Autodesk Inventor part; units mm, degrees
ref_plane "YZ Plane" through (0, 0, 0) normal (1, 0, 0) x (0, 1, 0)
ref_plane "XZ Plane" through (0, 0, 0) normal (0, 1, 0) x (-1, 0, 0)
ref_plane "XY Plane" through (0, 0, 0) normal (0, 0, 1) x (1, 0, 0)
sketch "Sketch1" plane through (0, 0, 0) normal (0, 0, 1) x (1, 0, 0)
  circle A0 centre (0, 0) radius 200
  line L0 (0, 187.7709) -> (15, 187.7709)
  line L1 (15, 187.7709) -> (15, 182.7709)
  line L2 (15, 182.7709) -> (50, 182.7709)
  line L3 (50, 182.7709) -> (50, 147.7709)
  line L4 (50, 147.7709) -> (-50, 147.7709)
  line L5 (-50, 147.7709) -> (-50, 182.7709)
  line L6 (-50, 182.7709) -> (-15, 182.7709)
  line L7 (-15, 182.7709) -> (-15, 187.7709)
  line L8 (-15, 187.7709) -> (0, 187.7709)
  line L9 (-162.6144, -93.8855) -> (-170.1144, -80.8951)
  line L10 (-170.1144, -80.8951) -> (-165.7843, -78.3951)
  line L11 (-165.7843, -78.3951) -> (-183.2843, -48.0842)
  line L12 (-183.2843, -48.0842) -> (-152.9734, -30.5842)
  line L13 (-152.9734, -30.5842) -> (-102.9734, -117.1867)
  line L14 (-102.9734, -117.1867) -> (-133.2843, -134.6867)
  line L15 (-133.2843, -134.6867) -> (-150.7843, -104.3758)
  line L16 (-150.7843, -104.3758) -> (-155.1144, -106.8758)
  line L17 (-155.1144, -106.8758) -> (-162.6144, -93.8855)
  line L18 (162.6144, -93.8855) -> (155.1144, -106.8758)
  line L19 (155.1144, -106.8758) -> (150.7843, -104.3758)
  line L20 (150.7843, -104.3758) -> (133.2843, -134.6867)
  line L21 (133.2843, -134.6867) -> (102.9734, -117.1867)
  line L22 (102.9734, -117.1867) -> (152.9734, -30.5842)
  line L23 (152.9734, -30.5842) -> (183.2843, -48.0842)
  line L24 (183.2843, -48.0842) -> (165.7843, -78.3951)
  line L25 (165.7843, -78.3951) -> (170.1144, -80.8951)
  line L26 (170.1144, -80.8951) -> (162.6144, -93.8855)
  line L27 (12.5, 183.7364) -> (12.5, 193.7364)
  line L28 (-173.6251, 83.379) -> (-162.3777, 105.706)
  line L29 (-162.3777, 105.706) -> (-153.4469, 101.2071)
  line L30 (-153.4469, 101.2071) -> (-164.6943, 78.88)
  line L31 (-164.6943, 78.88) -> (-173.6251, 83.379)
  line L32 (-181.8421, 26.8753) -> (-182.5998, 1.8868)
  line L33 (-192.5952, 2.1899) -> (-191.8375, 27.1784)
  line L34 (-182.5998, 1.8868) -> (-192.5952, 2.1899)
  line L35 (-191.8375, 27.1784) -> (-181.8421, 26.8753)
  line L36 (-115.9276, 141.0924) -> (-122.1203, 148.9442)
  line L37 (-96.2982, 156.5742) -> (-115.9276, 141.0924)
  line L38 (-102.4909, 164.426) -> (-96.2982, 156.5742)
  line L39 (-122.1203, 148.9442) -> (-102.4909, 164.426)
  line L40 (72.3815, -179.7253) -> (67.6463, -170.9175)
  line L41 (67.6463, -170.9175) -> (89.6659, -159.0795)
  line L42 (94.4011, -167.8873) -> (72.3815, -179.7253)
  line L43 (89.6659, -159.0795) -> (94.4011, -167.8873)
  line L44 (14.035, -182.0694) -> (14.6042, -192.0532)
  line L45 (-10.9244, -183.4924) -> (14.035, -182.0694)
  line L46 (-10.3552, -193.4762) -> (-10.9244, -183.4924)
  line L47 (14.6042, -192.0532) -> (-10.3552, -193.4762)
  line L48 (-64.2258, -170.9424) -> (-67.9293, -180.2313)
  line L49 (-87.4482, -161.6838) -> (-64.2258, -170.9424)
  line L50 (-67.9293, -180.2313) -> (-91.1516, -170.9727)
  line L51 (-91.1516, -170.9727) -> (-87.4482, -161.6838)
  line L52 (119.4559, 152.5469) -> (114.1957, 144.0422)
  line L53 (114.1957, 144.0422) -> (92.9339, 157.1927)
  line L54 (98.1941, 165.6974) -> (119.4559, 152.5469)
  line L55 (92.9339, 157.1927) -> (98.1941, 165.6974)
  line L56 (150.6592, 103.1894) -> (159.0209, 108.6742)
  line L57 (164.3713, 82.2854) -> (150.6592, 103.1894)
  line L58 (172.7329, 87.7702) -> (164.3713, 82.2854)
  line L59 (159.0209, 108.6742) -> (172.7329, 87.7702)
  line L60 (180.1534, 29.85) -> (190.0496, 31.2872)
  line L61 (183.7463, 5.1095) -> (180.1534, 29.85)
  line L62 (190.0496, 31.2872) -> (193.6425, 6.5467)
  line L63 (193.6425, 6.5467) -> (183.7463, 5.1095)
  point P0 (-163.536, 92.293)
  point P1 (-187.2187, 14.5326)
  point P2 (-109.2092, 152.7592)
  point P3 (81.0237, -169.4024)
  point P4 (1.8399, -187.7728)
  point P5 (-77.6887, -170.9575)
  point P6 (106.1949, 154.8698)
  point P7 (161.6961, 95.4798)
  point P8 (186.8979, 18.1984)
  dimension "d12" = 360
  dimension "d28" = 25
  dimension "d32" = 25
  dimension "d36" = 360
extrude "Extrusion1" add sketch "Sketch1" along normal blind 1.5
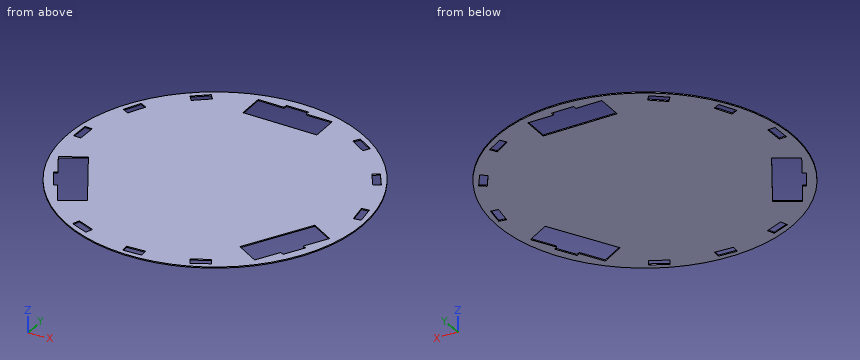
Could you check a few things on this model? Use its own coordinates, in mm. Coordinates: 2 decimals unless noted, no trailing zeros. Order: outer loops, then holes, each group sorted by start corner. A loop starts at its lowest first (then second) coordinate and runs counter-clockwise, first axis right, second up.
Q1. Please list where these lines run through material, in increasing order: L1, parallel to X at y = 84.5, z = 0.1; L2, parallel to X at y = -44, z = 0.9; L3, parallel to Y at x = 108.5, z = 0.95.
Q2. Suppose I cut it at B-B on y = -43. Please give me the cut outline in (x, z).
Q3. Suppose I cut it at C-C on x = 40. Please give me the cut outline in (y, z).
Q4. Will this pin go through, and if not, where does the flat tip stop? pin 1 (0.8 mm diameter, centred on y = 169.5, z = 0.5, fed in from +X).
Q5. Suppose I cut it at D-D on z = 0.5. Give the number of separate pieces and of enclosed holes in the cut face, and give its area (3 significant figures).
Q6. Suppose I cut it at A-A on x = -33.5. Please give me the cut outline in (y, z), and give its area (3 significant figures).
Answer:
1. L1: x = -181.27 to -173.06, -161.86 to 162.92, 167.75 to 181.27
1. L2: x = -195.1 to -176.21, -145.23 to 145.23, 176.21 to 195.1
1. L3: y = -168.01 to -120.38, -107.61 to 147.57, 159.32 to 168.01
2. outline: (-195.32, 0) - (-174.48, 0) - (-174.48, 1.5) - (-195.32, 1.5) - close; (-145.81, 0) - (145.81, 0) - (145.81, 1.5) - (-145.81, 1.5) - close; (174.48, 0) - (195.32, 0) - (195.32, 1.5) - (174.48, 1.5) - close
3. outline: (-195.96, 0) - (147.77, 0) - (147.77, 1.5) - (-195.96, 1.5) - close; (182.77, 0) - (195.96, 0) - (195.96, 1.5) - (182.77, 1.5) - close
4. pin 1: stops at x = 106.8
5. separate pieces: 1
5. enclosed holes: 12
5. area: 112,000 mm2
6. outline: (-197.17, 0) - (147.77, 0) - (147.77, 1.5) - (-197.17, 1.5) - close; (182.77, 0) - (197.17, 0) - (197.17, 1.5) - (182.77, 1.5) - close
6. area: 539 mm2
